Autodesk Inventor part; units mm, degrees
ref_plane "YZ Plane" through (0, 0, 0) normal (1, 0, 0) x (0, 1, 0)
ref_plane "XZ Plane" through (0, 0, 0) normal (0, 1, 0) x (-1, 0, 0)
ref_plane "XY Plane" through (0, 0, 0) normal (0, 0, 1) x (1, 0, 0)
sketch "Sketch1" plane through (0, 0, 0) normal (0, 0, 1) x (1, 0, 0)
  line L0 (0, 0) -> (31.75, 0)
  line L1 (31.75, 0) -> (31.75, -18.415)
  line L2 (31.75, -18.415) -> (0, -18.415)
  line L3 (0, -18.415) -> (0, 0)
  dimension "d0" = 31.75
  dimension "d1" = 18.415
extrude "Extrusion1" add sketch "Sketch1" along normal blind 6.35
sketch "Sketch2" plane through (0, 0, 0) normal (0, 1, 0) x (1, 0, 0)
  line L0 (2.54, -1.5875) -> (29.21, -1.5875)
  line L1 (29.21, -1.5875) -> (29.21, -4.7625)
  line L2 (29.21, -4.7625) -> (2.54, -4.7625)
  line L3 (2.54, -4.7625) -> (2.54, -1.5875)
  line L4 (0, 0) -> (0, -6.35)
  line L5 (31.75, -6.35) -> (0, -6.35)
  dimension "d4" = 26.67
  dimension "d5" = 2.54
  dimension "d6" = 3.175
  dimension "d7" = 1.5875
extrude "Extrusion2" cut sketch "Sketch2" against normal blind 16.51
sketch "Sketch3" plane through (29.21, 0, 4.7625) normal (0, 0, -1) x (-1, 0, 0)
  line L0 (1.27, 0) -> (25.4, 0)
  line L1 (25.4, 0) -> (25.4, -15.24)
  line L2 (25.4, -15.24) -> (1.27, -15.24)
  line L3 (1.27, -15.24) -> (1.27, 0)
  line L4 (26.67, -16.51) -> (0, -16.51)
  line L5 (26.67, 0) -> (26.67, -16.51)
  line L6 (0, 0) -> (0, -16.51)
  line L7 (0, 0) -> (26.67, 0)
  point P0 (29.21, 0)
  dimension "d10" = 1.27
  dimension "d11" = 1.27
  dimension "d12" = 1.27
  dimension "d13" = 0
extrude "Extrusion3" cut sketch "Sketch3" against normal blind 16.51 contours L0 L1 L2 L3
sketch "Sketch4" plane through (0, -18.415, 0) normal (0, -1, 0) x (1, 0, 0)
  circle A0 centre (1.905, 3.175) radius 1.5621
  circle A1 centre (29.845, 3.175) radius 1.5621
  line L0 (0, 6.35) -> (31.75, 6.35)
  line L1 (0, 0) -> (0, 6.35)
  dimension "d16" = 3.1242
  dimension "d17" = 3.1242
  dimension "d18" = 3.175
  dimension "d19" = 3.175
  dimension "d20" = 27.94
  dimension "d21" = 1.905
extrude "Extrusion4" add sketch "Sketch4" along normal blind 2.54
properties part number "CameraMount" material "ABS Plastic"
Verification items for the finished model (mm, model axes). A direction names the side the tool comes from. Round coordinates to 2 decimals unless told otherwise and drop trailing zeros. Order: outer loops, then holes, each group sorted by start corner. A loop starts at its lowest first (then second) coordinate and runs counter-clockwise, first axis right, second up.
1) Tool access check on faces 4 (the cylindrical face through (0.754, -19.667, 2.119)), 5 (the flat face through (2.54, -8, 3)), 6 (the flat face through (16, -15.24, 6)). Record the directions out of +Z, -Z, +X, -X, +Y, -Y that give a thin tool (end or side, any length) a straight path to the whole face; none if there is none.
Geometry says:
face 4: -Y
face 5: +Y
face 6: +Z, +Y
2) Depth check by flat-ended pin: pin 1 (1 mm diameter, centred on x = 17.5, z = 3.5, fed in from +Y); pin 2 (1.9 mm diameter, centred on x = 19.5, z = 4, fed in from -Y) (3 decimals); pin 3 (0.8 mm diameter, centred on x = 13.5, z = 5, fed in from +Y). Enter the tip coordinate at first touch or a pass-through.
Geometry says:
pin 1: stops at y = -16.51
pin 2: stops at y = -18.415
pin 3: stops at y = -15.24
3) Cross-section at B-B, the plane z = 5.75. Record the cut outline in (x, y) (3 decimals), plus the area to 3 significant figures.
Geometry says:
outline: (0, -18.415) - (31.75, -18.415) - (31.75, 0) - (27.94, 0) - (27.94, -15.24) - (3.81, -15.24) - (3.81, 0) - (0, 0) - close
area: 217 mm2
4) Cross-section at D-D, the plane z = 3.5. Record the cut outline in (x, y) (3 decimals), plus the area to 3 significant figures.
Geometry says:
outline: (0, -18.415) - (0.377, -18.415) - (0.377, -20.955) - (3.433, -20.955) - (3.433, -18.415) - (28.317, -18.415) - (28.317, -20.955) - (31.373, -20.955) - (31.373, -18.415) - (31.75, -18.415) - (31.75, 0) - (29.21, 0) - (29.21, -16.51) - (2.54, -16.51) - (2.54, 0) - (0, 0) - close
area: 160 mm2
5) Draft check along Z on faces 1 (the flat face through (16, -16, 6.35)), 2 (the cylindrical face through (28.284, -19.667, 3.106)), 3 (the flat face through (16, -16, 4.762)). Enter one of: +Z half, -Z half, draft (parallel to the pull), parting line (faces both ways), or undercut.
Geometry says:
face 1: +Z half
face 2: parting line
face 3: undercut
6) Cross-section at A-A, the plane y = -5. Record the cut outline in (x, z).
Geometry says:
outline: (0, 0) - (31.75, 0) - (31.75, 6.35) - (27.94, 6.35) - (27.94, 4.76) - (29.21, 4.76) - (29.21, 1.59) - (2.54, 1.59) - (2.54, 4.76) - (3.81, 4.76) - (3.81, 6.35) - (0, 6.35) - close
7) Material ranges on line 1 (Z direction, x = 3.5, y = -15.75); line 2 (X direction, y = -15, z = 6.25); line 3 (X direction, y = -15, z = 4.5), recorded low to high.
Geometry says:
line 1: z = 0 to 1.59, 4.76 to 6.35
line 2: x = 0 to 3.81, 27.94 to 31.75
line 3: x = 0 to 2.54, 29.21 to 31.75
